Read the model definition and answer for the solid it produces. Units are mm, in the model's axes. Coordinates: 2 decimals unless noted, no trailing zeros. Order: outer loops, then holes, each group sorted by start corner. A loop starts at its lowest first (then second) coordinate and runs counter-clockwise, first axis right, second up. Notation, with made-up numbers: M 89.25,56 L 135.25,56 A11 cw 135.25,63 Z; hole C 15,77.25 d3. An arc over 180 degrees is marked long. Write each question's results on one line, items separated by ' | '.
```python
from build123d import *

# Parameters (mm, degrees)
F1_DEPTH = 25
F3_DEPTH = 25


with BuildPart() as f1:
    # F0 (on Right) → F1 (new body)
    with BuildSketch(Plane.YZ):
        Polygon((0, 10), (0, 0), (0, -15), (2, -15), (2, 2), (2, 10), align=None)
    extrude(amount=F1_DEPTH)

    # F2 (on face) → F3 (cut)
    with BuildSketch(Plane(origin=(0, 2, 0), x_dir=(-1, 0, 0), z_dir=(0, 1, 0))):
        with BuildLine():
            Line((-15.875, 3), (-15.875, 7))
            ThreePointArc((-15.875, 7), (-17.5, 8.625), (-19.125, 7))
            Line((-19.125, 7), (-19.125, 3))
            ThreePointArc((-19.125, 3), (-17.5, 1.375), (-15.875, 3))
        make_face()
        with BuildLine():
            Line((-5.875, 3), (-5.875, 7))
            ThreePointArc((-5.875, 7), (-7.5, 8.625), (-9.125, 7))
            Line((-9.125, 7), (-9.125, 3))
            ThreePointArc((-9.125, 3), (-7.5, 1.375), (-5.875, 3))
        make_face()
    extrude(amount=-F3_DEPTH, mode=Mode.SUBTRACT)


solid = f1.part
```
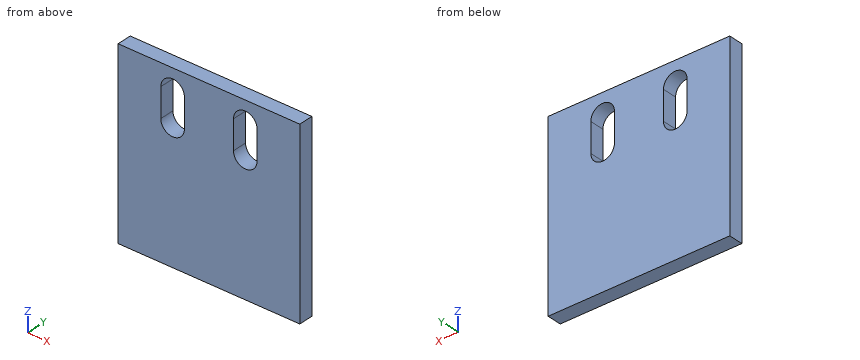
(1) The part is cut by section C-C, the plane y = 0.5. Write down the section's boundary in (x, z) (3 decimals), then the cut area to 3 significant figures.
Conclusion:
outline: M 0,-15 L 25,-15 L 25,10 L 0,10 Z; hole M 5.875,3 A1.625 ccw 9.125,3 L 9.125,7 A1.625 ccw 5.875,7 Z; hole M 15.875,3 A1.625 ccw 19.125,3 L 19.125,7 A1.625 ccw 15.875,7 Z | area: 582 mm²
(2) Given pin 1 (1 mm diameter, centred on y = 0, z = 4, fed in from -X), flat-ended and moving along its own axis, determine where the tip first touches the part or whether it passes through.
Conclusion:
pin 1: x = 0
(3) Straight lines are drawn through the part: line 1 (X direction, y = 0.1, z = 7) (3 decimals); line 2 (Z direction, x = 8.25, y = 0.3); line 3 (Z direction, x = 7.75, y = 1.9). For each, find the intervals that lie inside material, in ascending order.
Conclusion:
line 1: 0 to 5.875, 9.125 to 15.875, 19.125 to 25 | line 2: -15 to 1.56, 8.44 to 10 | line 3: -15 to 1.39, 8.61 to 10
(4) The part is cut by section D-D, the plane x = 17.25. Write down the section's boundary in (y, z), then the cut area to 3 significant figures.
Conclusion:
outline: M 0,-15 L 2,-15 L 2,1.39 L 0,1.39 Z; M 0,8.61 L 2,8.61 L 2,10 L 0,10 Z | area: 35.6 mm²
(5) The part is cut by section B-B, the plane z = 5.75. Write down the section's boundary in (x, y) (3 decimals), then the cut area to 3 significant figures.
Conclusion:
outline: M 0,0 L 5.875,0 L 5.875,2 L 0,2 Z; M 9.125,0 L 15.875,0 L 15.875,2 L 9.125,2 Z; M 19.125,0 L 25,0 L 25,2 L 19.125,2 Z | area: 37.0 mm²
(6) The part is cut by section A-A, the plane x = 7.5. Write down the section's boundary in (y, z) (3 decimals).
Conclusion:
outline: M 0,-15 L 2,-15 L 2,1.375 L 0,1.375 Z; M 0,8.625 L 2,8.625 L 2,10 L 0,10 Z
